Part model, mm, in its own coordinate system. Face numbers are marked on the shaded views. A direction names the side the tool comes from. Give positions to 0.01 mm unless a question says otherwise; leave off trailing zeros. Loops run counter-clockwise (first coordinate to the right, second up) from the corner with the lowest first, then second, coordinate; pieces in that order, holes last. Notation, with made-up numbers: (40.5, -10) -> (82.5, -10) arc R13 cw to (82.5, 11) -> close; hole circle Ø6 at (52.25, 83.5). An arc over 180 degrees is marked (long way). Write item = value, one per line.
from build123d import *

# Parameters (mm, degrees)
F1_DEPTH = 63.5
F0_W     = 25.4
F0_H     = 19.05
F2_DEPTH = 25.4
F3_DEPTH = 7.9375


with BuildPart() as f1:
    # F0 (on Front) → F1 (new body, symmetric)
    with BuildSketch(Plane.XZ):
        Polygon((41.275, -9.525), (41.275, 9.525), (22.225, 9.525), (-41.275, 9.525), (-41.275, -9.525), align=None)
    extrude(amount=F1_DEPTH, both=True)

    # F0 (on Front) → F2 (join, symmetric)
    with BuildSketch(Plane.XZ):
        with BuildLine():
            Line((22.225, 9.525), (41.275, 9.525))
            Line((41.275, 9.525), (41.275, 27.0002))
            ThreePointArc((41.275, 27.0002), (45.9246798487, 38.2255201513), (57.15, 42.8752))
            Line((57.15, 42.8752), (60.325, 42.8752))
            Line((60.325, 42.8752), (60.325, 61.9252))
            Line((60.325, 61.9252), (57.15, 61.9252))
            add(Edge.make_bspline(
                [(55.3448990391, 61.8785204229), (55.9525265065, 61.8965004125), (56.5543434747, 61.9120279552), (57.15, 61.9252)],
                knots=[109.7015046992, 109.7015046992, 109.7015046992, 109.7015046992, 111.5045361635, 111.5045361635, 111.5045361635, 111.5045361635], degree=3))
            ThreePointArc((55.3448990391, 61.8785204229), (31.8241359865, 51.0492381714), (22.225, 27.0002))
            Line((22.225, 27.0002), (22.225, 9.525))
        make_face()
        with Locations((73.025, 52.4002)):
            Rectangle(F0_W, F0_H)
    extrude(amount=F2_DEPTH, both=True)

    # F0 (on Front) → F3 (join, symmetric)
    with BuildSketch(Plane.XZ):
        with BuildLine():
            Line((-41.275, 9.525), (22.225, 9.525))
            Line((22.225, 9.525), (22.225, 27.0002))
            ThreePointArc((22.225, 27.0002), (31.8241359865, 51.0492381714), (55.3448990391, 61.8785204229))
            add(Edge.make_bspline(
                [(-41.275, 9.525), (-40.1042120828, 50.6120289683), (18.3751351779, 60.7845672918), (55.3448990391, 61.8785204229)],
                knots=[0, 0, 0, 0, 109.7015046992, 109.7015046992, 109.7015046992, 109.7015046992], degree=3))
        make_face()
    extrude(amount=F3_DEPTH, both=True)


solid = f1.part
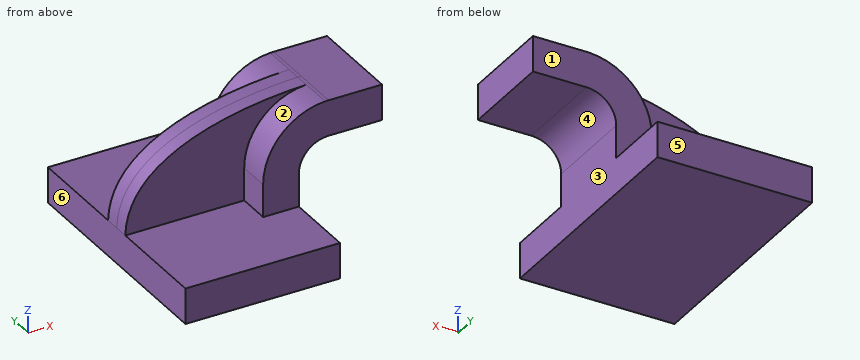
1) Drill centre lines: line 1 along Y through (x, z) = (13.5, 12.5); line 2 along Y through (x, z) = (36, 20.5); line 3 along X through (y, z) = (-23.5, 27) (3 decimals). Where is each one in solid material? Low to high. Write a range as [from, to].
Resolved:
line_1 = [-7.94, 7.94]
line_2 = [-25.4, 25.4]
line_3 = [22.225, 41.275]
2) Slice it at A-A, the plane y = 55. List the corners of the cut face in (x, z) (3 decimals).
Resolved:
outline = (-41.275, -9.525) -> (41.275, -9.525) -> (41.275, 9.525) -> (-41.275, 9.525) -> close
3) Drop flat-ended pins along their axis: P1, Ø8.5, axis at x = 68, y = 12, coming from the -Z side; P2, Ø16.5, axis at x = -16, y = -40, coming from the +Z side (3 decimals); P3, Ø1.5, axis at x = -11.5, z = 20, coming from the +Y side. Give the stop position or say it passes through.
Resolved:
P1 = 42.88
P2 = 9.525
P3 = 7.94
4) Pull direction X, two halves, no side cores. Call the marked faces 4, 5 and 6: pulls with the +X half, pulls with the -X half, needs draft (parallel to the pull), parting line crosses it, or undercut.
Resolved:
face_4 = pulls with the +X half
face_5 = needs draft
face_6 = pulls with the -X half
5) Slice it at B-B, the plane z = 2. List the corners of the cut face in (x, y) (3 decimals).
Resolved:
outline = (-41.275, -63.5) -> (41.275, -63.5) -> (41.275, 63.5) -> (-41.275, 63.5) -> close
6) Which spindle directions (+Z, -Z, +X, -X, +Y, -Y) get a long thin tool onto all of the face, cutting with end or side? Do the marked faces 1, 2 and 3. Say none if no direction does.
Resolved:
face_1 = +Z, +X, -X, +Y
face_2 = +Z, -X, -Y
face_3 = -Z, +X, +Y, -Y
